Input: dimensioned drawing with shaded views. Units: mm. Origin: part minimum x, y, z. Give positions to 0.01 mm unless a question says otherwise; leave off trailing zeros. Loops run counter-clockwise (first coordinate to the right, second up) from the corner with the lowest first, then second, coordinate; pieces in that order, holes last. Notation, with made-up numbers: (-24, -12) -> (2, -12) arc R33 ccw to (2, 23) -> close; hole circle Ø8 at (-7, 38.5). An arc over 180 degrees is marked (long way). One line per question, with ' | ' between items. Start each with the question number.
Item 1: Material intervals for line 1 along Z through (x, y) = (5.9, 6.75) (1 decimal); line 2 along Z through (x, y) = (6.75, 5.25); line 3 along X through (y, z) = (7.5, 4.5), sorted ascending. Write a range as [from, to].
Item 2: Section D-D on z = 9. Return loops of the section in (x, y) (1 decimal).
Item 3: Mould query, pull axis X, two halves, no side actions, for the marked faces 1, 2 and 3. Classes: released by +X, released by -X, zero draft, split by the parting line, or undercut.
Item 4: Pin query (flat end, axial travel): P1, Ø5, axis at x = 5.9, z = 5.4, coming from the +Y side; P2, Ø2, axis at x = 8, y = 3.5, coming from the +Z side; P3, Ø1.5, axis at y = 1, z = 2.5, coming from the +X side (1 decimal). Return the tip coordinate at first contact, or that it passes through.
Item 5: Section B-B on z = 5.4. Return loops of the section in (x, y) (1 decimal).
Item 6: Section A-A on x = 5.9. Return loops of the section in (y, z) (1 decimal).
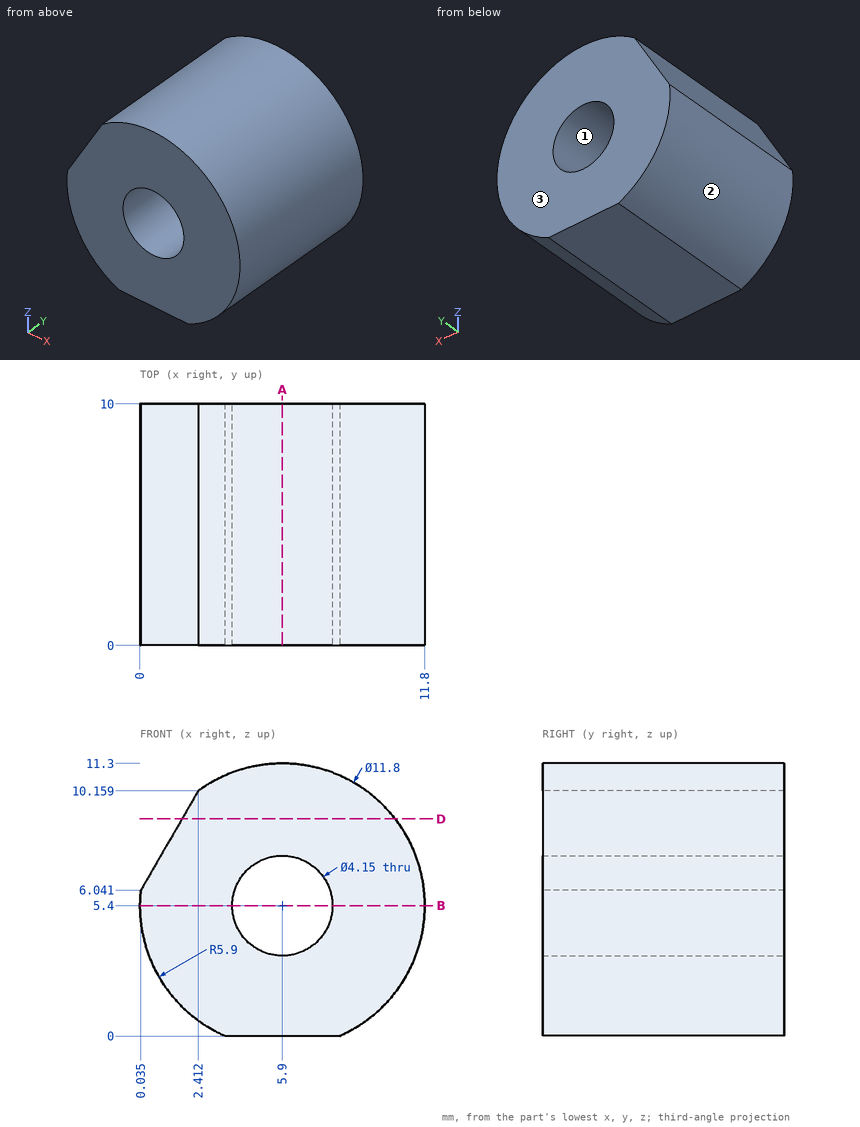
Result sheet:
1) line 1: z = [0, 3.3], [7.5, 11.3] | line 2: z = [0, 3.51], [7.29, 11.24] | line 3: x = [0.07, 4.03], [7.77, 11.73]
2) outline: (1.7, 0) -> (10.6, 0) -> (10.6, 10) -> (1.7, 10) -> close
3) face 1: undercut | face 2: released by -X | face 3: zero draft
4) P1: stops at y = 10 | P2: stops at z = 11.2 | P3: stops at x = 11.4
5) outline: (0, 0) -> (3.8, 0) -> (3.8, 10) -> (0, 10) -> close; (8, 0) -> (11.8, 0) -> (11.8, 10) -> (8, 10) -> close
6) outline: (0, 0) -> (10, 0) -> (10, 3.3) -> (0, 3.3) -> close; (0, 7.5) -> (10, 7.5) -> (10, 11.3) -> (0, 11.3) -> close
